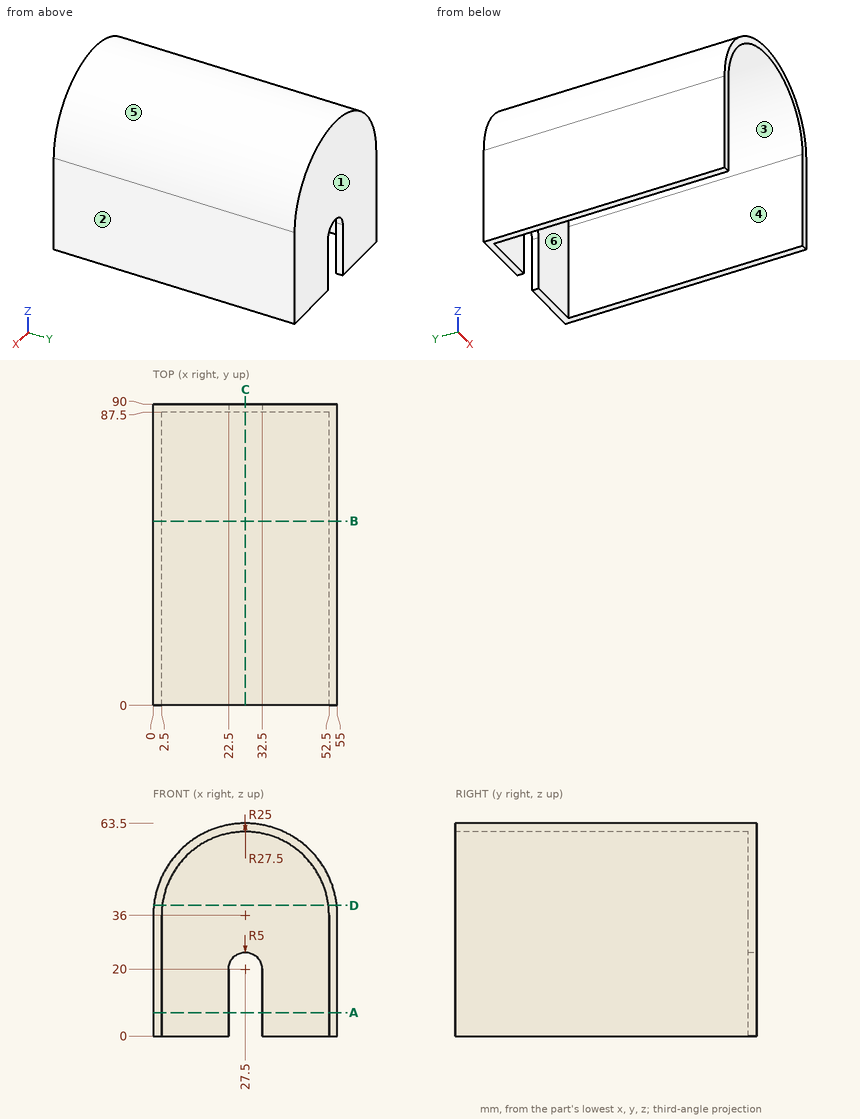
Geometry: see drawing. Coordinates: mm, zero at the bounding-box minimum. A direction names the side the tool comes from. Give positions to 0.01 mm unless a question says otherwise; leave off trailing zeros. Write each loop counter-clockwise with the first axis right and the second up, starting at its lowest first coordinate (ties: lowest second). Pieces come first, ordered by that corner, then holes. Notation, with made-up numbers: (21, 43.25) - (44, 43.25) arc R21 ccw to (44, 50.25) - close; hole circle Ø5 at (74, -35). An arc over 180 degrees is marked (long way). Return JSON: item names as keys, results as strings. Group by question number.
1) Section D-D on z = 39. Return the cut outline in (x, y).
2) Line query: line 1 (X direction, y = 59, z = 20); line 2 (Y direction, x = 22, z = 39); line 3 (X direction, y = 14, z = 45.5). Output: solid intervals per line, ascending.
3) Mould query, pull axis X, two halves, no side actions, for the marked faces 1, 2, 3 and 4. Classes: released by +X, released by -X, zero draft, split by the parting line, or undercut.
4) Section C-C on x = 27.5. Return the cut outline in (y, z), plus the area to 3 significant figures.
5) Section B-B on y = 55. Return the cut outline in (x, z), plus the area to 3 significant figures.
6) Section A-A on z = 7. Return the cut outline in (x, y), plus the area to 3 significant figures.
7) First-contact query: P1, Ø4, axis at x = 46.5, y = 51.5, coming from the -Z side; P2, Ø10, axis at x = 46.5, y = 65.5, coming from the +Z side; P3, Ø8, axis at y = 69.5, z = 45, coming from the +X side. Flat tips, straight axial feed; report the tip coordinate or a pass-through.
8) Set-up query: the marked faces 5 and 6. Return all of +Z, -Z, +X, -X, +Y, -Y with unobstructed straight access to the full face (end or side cutting, diameter ignored); none if empty.
Filled in:
{
 "1": {"outline": "(0.16, 0) - (2.68, 0) - (2.68, 87.5) - (52.32, 87.5) - (52.32, 0) - (54.84, 0) - (54.84, 90) - (0.16, 90) - close"},
 "2": {"line 1": "x = 0 to 2.5, 52.5 to 55", "line 2": "y = 87.5 to 90", "line 3": "x = 1.69 to 4.38, 50.62 to 53.31"},
 "3": {"face 1": "zero draft", "face 2": "released by +X", "face 3": "undercut", "face 4": "undercut"},
 "4": {"outline": "(0, 61) - (87.5, 61) - (87.5, 25) - (90, 25) - (90, 63.5) - (0, 63.5) - close", "area": "315 mm^2"},
 "5": {"outline": "(0, 0) - (2.5, 0) - (2.5, 36) arc R25 cw to (52.5, 36) - (52.5, 0) - (55, 0) - (55, 36) arc R27.5 ccw to (0, 36) - close", "area": "386 mm^2"},
 "6": {"outline": "(0, 0) - (2.5, 0) - (2.5, 87.5) - (22.5, 87.5) - (22.5, 90) - (0, 90) - close; (32.5, 87.5) - (52.5, 87.5) - (52.5, 0) - (55, 0) - (55, 90) - (32.5, 90) - close", "area": "550 mm^2"},
 "7": {"P1": "stops at z = 49.56", "P2": "stops at z = 59.67", "P3": "stops at x = 54.54"},
 "8": {"face 5": "+Z, +Y, -Y", "face 6": "-Z, -Y"}
}
